Read the model definition and answer for the solid it produces. Units are mm, in the model's axes. Coordinates: 2 decimals unless noted, no trailing zeros. Order: outer loops, then holes, each group sorted by start corner. A loop starts at its lowest first (then second) coordinate and runs counter-clockwise, first axis right, second up. Notation, with made-up numbers: (72, 25) - (115, 25) arc R18 cw to (115, 38) - close; hole circle Ø2 at (-2.75, 51.5). An arc over 180 degrees is marked (long way). Write item = value, one per line.
from build123d import *

# Parameters (mm, degrees)
SKETCH_4_R          = 4
EXTRUDE_3_DEPTH     = 20
CUT_EXTRUDE_1_REACH = 174.818
SKETCH_5_R          = 4


with BuildPart() as part:
    # 草图4 → 凸台-拉伸3 (new body)
    with BuildSketch(Plane.XY):
        Polygon((-7, 6), (15, 6), (15, -6), (15, -171), (-7, -171), (-7, -6), align=None)
        Circle(SKETCH_4_R, mode=Mode.SUBTRACT)
    extrude(amount=EXTRUDE_3_DEPTH)

    # 草图5 → 切除-拉伸1 (cut, up to next)
    with BuildSketch(Plane.XY.offset(20), mode=Mode.PRIVATE) as cut_extrude_1_sk1:
        with Locations((4, -131)):
            Circle(SKETCH_5_R)
    cut_extrude_1_tool1 = extrude(cut_extrude_1_sk1.sketch, amount=-CUT_EXTRUDE_1_REACH, mode=Mode.PRIVATE) & part.part
    # 草图5 → 切除-拉伸1 (cut, up to next)
    with BuildSketch(Plane.XY.offset(20), mode=Mode.PRIVATE) as cut_extrude_1_sk2:
        with Locations((4, -156)):
            Circle(SKETCH_5_R)
    cut_extrude_1_tool2 = extrude(cut_extrude_1_sk2.sketch, amount=-CUT_EXTRUDE_1_REACH, mode=Mode.PRIVATE) & part.part
    add(cut_extrude_1_tool1.solids().sort_by_distance((4, -131, 20))[0], mode=Mode.SUBTRACT)
    add(cut_extrude_1_tool2.solids().sort_by_distance((4, -156, 20))[0], mode=Mode.SUBTRACT)


solid = part.part
1) Flat-ended cylindrical pins translate along their axes: pin 1 Ø7 at (x, y) = (4, -131) entering from +Z; pin 2 Ø5 at (x, y) = (11, -130) entering from -Z. Find the tip coordinate at first contact, or state that the pin passes through.
Returned:
pin_1 = through
pin_2 = 0
2) The part is cut by section A-A (y = -131). Determine the outline of the cut face in (x, z), and give its area (3 significant figures).
Returned:
outline = (-7, 0) - (0, 0) - (0, 20) - (-7, 20) - close; (8, 0) - (15, 0) - (15, 20) - (8, 20) - close
area = 280 mm^2
3) The part is cut by section B-B (z = 16.75). Determine the outline of the cut face in (x, y).
Returned:
outline = (-7, -171) - (15, -171) - (15, 6) - (-7, 6) - close; hole circle Ø8 at (0, 0); hole circle Ø8 at (4, -156); hole circle Ø8 at (4, -131)
4) Straight lines are drawn through the part: line 1 along Y through (x, z) = (0.75, 11.25); line 2 along Y through (x, z) = (4.75, 10.75); line 3 along X through (y, z) = (-159.5, 17.5). For each, find the intervals that lie inside material, in ascending order. Write a range as from..to.
Returned:
line_1 = -171..-158.33, -153.67..-133.33, -128.67..-3.93, 3.93..6
line_2 = -171..-159.93, -152.07..-134.93, -127.07..6
line_3 = -7..2.06, 5.94..15
5) Determine the mould class of faces 1 (the face through (-7, -81, 10)), 2 (the face through (-0.867, -3.905, 9.86)), 3 (the face through (15, -84, 10)) for opening direction X: pulls with the +X half, pulls with the -X half, needs draft (parallel to the pull), parting line crosses it, or undercut.
Returned:
face_1 = pulls with the -X half
face_2 = undercut
face_3 = pulls with the +X half
